Study the drawing (mm; zero at the part's minimum x, y, z) and answer. Round coordinates to 2 decimals unless told otherwise and drop trailing zeros. Write each loop counter-clockwise with the first axis right and the second up, starting at its lowest first coordinate (ties: lowest second). Pieces come first, ordered by that corner, then holes.
(1) A cutting plane is placed at D-D, the plane z = 36.5. Give the vertices of the cut face in (x, y), and give its area (3 significant figures).
(2) The mould has two halves that part along Z. Classify the marked faces 1, 2 and 3: +Z half, -Z half, draft (parallel to the pull), parting line (faces both ways), or undercut.
(3) A cutting plane is placed at A-A, the plane z = 10.5. Give the vertices of the cut face in (x, y), and give its area (3 significant figures).
(4) A cutting plane is placed at C-C, the plane x = 156. Give the vertices of the cut face in (y, z), and give its area (3 significant figures).
(5) A cutting plane is placed at B-B, the plane y = 28. Give the vertices of the cut face in (x, z), and give its area (3 significant figures).
(6) Find the intervals of material crossed by probe 1 along Y at (x, z) = (295, 18.5); probe 2 along Z at (x, y) = (258.5, 19); probe 3 along X at (y, z) = (3, 14), in increasing order.
(7) Each of these flat-tipped pins is pushed along its axis until it touches: pin 1 Ø5 at (x, y) = (187.5, 11.5) entering from +Z; pin 2 Ø7 at (x, z) = (143, 29.5) entering from -Y. Where does it stop, or does it pass through?
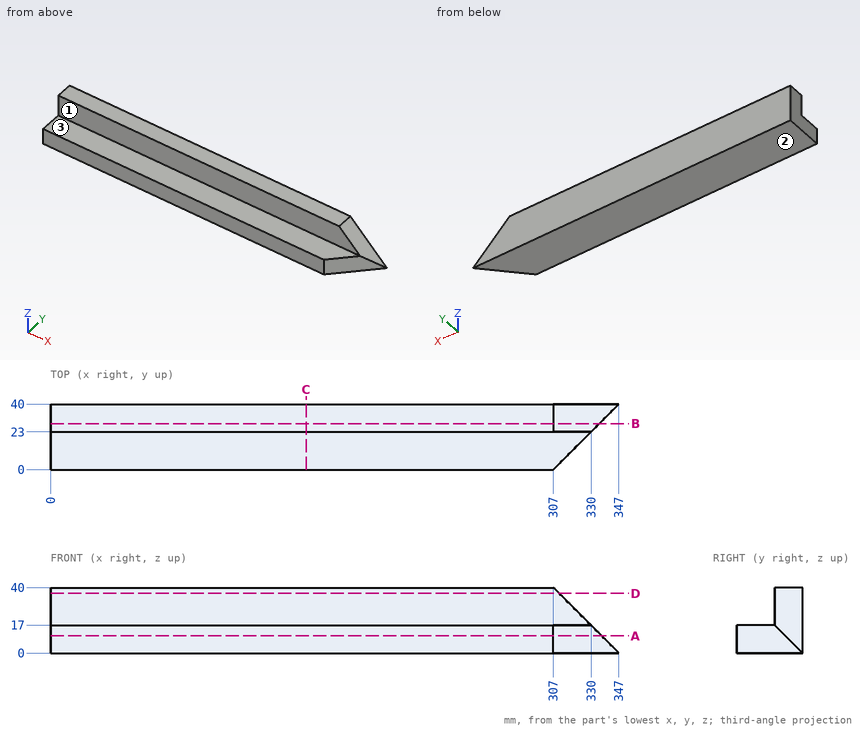
Solutions:
1. outline: (0, 23) - (310.5, 23) - (310.5, 40) - (0, 40) - close
1. area: 5,280 mm2
2. face 1: draft
2. face 2: -Z half
2. face 3: +Z half
3. outline: (0, 0) - (307, 0) - (336.5, 29.5) - (336.5, 40) - (0, 40) - close
3. area: 13,000 mm2
4. outline: (0, 0) - (40, 0) - (40, 40) - (23, 40) - (23, 17) - (0, 17) - close
4. area: 1,070 mm2
5. outline: (0, 0) - (335, 0) - (335, 12) - (307, 40) - (0, 40) - close
5. area: 13,000 mm2
6. probe 1: y = 23 to 40
6. probe 2: z = 0 to 17
6. probe 3: x = 0 to 310
7. pin 1: stops at z = 17
7. pin 2: stops at y = 23
